Verification items for the finished model (mm, model axes). A direction names the side the tool comes from. Give positions to 0.01 mm unless a question says otherwise; leave off trailing zeros. Loops run counter-clockwise (first coordinate to the right, second up) from the corner with the lowest first, then second, coordinate; pieces in that order, holes last. Notation, with made-up numbers: (68, -22.75) -> (106, -22.75) arc R19 ccw to (106, -14.75) -> close; hole circle Ø7 at (-17.5, 3.5). An arc over 180 degrees is marked (long way). Answer in a Markdown table with one row per item. Add a question column.
Q1. Gauge pin test, flat ends, axial feed: P1, Ø1.5, axis at x = -2.5, y = 0.5, coming from the -Z side; P2, Ø1, axis at x = -10.5, z = 3.5, coming from the -Y side; P3, Ø1.5, axis at x = -10, z = 2, coming from the +Y side; P4, Ø2, axis at x = -14, z = 1.5, coming from the -Y side. Record the tip position at first contact, or that the pin passes through.
Q2. Material ranges on probe 1 along Z at (x, y) = (-2.5, 2.15); probe 2 along X at (y, z) = (-1.7, 3.5); probe 3 along Y at (x, z) = (-16, 0.7), recorded low to high.
Q3. Section check D-D on z = 0.9. Enter the section's corners in (x, y), and give its area (3 significant figures).
Q4. Section check B-B on y = 0.9. Enter the section's corners in (x, z), and give its area (3 significant figures).
Q5. Section check C-C on z = 3.1. Enter the section's corners in (x, y), and give its area (3 significant figures).
Q6. Release check for a two-part mould opening along X. For faces 3 (the face through (-8.35, -2.08, 0.99)), 4 (the face through (-16.37, 0.37, 0.99)), 5 (the face through (0, -2, 2)), 6 (the face through (-9, 0, 2)) record: pulls with the +X half, pulls with the -X half, needs draft (parallel to the pull), parting line crosses it, or undercut.
Q7. Section check A-A on x = 0. Enter the section's corners in (y, z), and give its area (3 significant figures).
Q8. Set-up check for faces 1 (the face through (2.77, -1.15, 2.42)), 2 (the face through (-17.25, 0.06, 0.99)): record each of +Z, -Z, +X, -X, +Y, -Y from which the full face is reachable in a straight line by a thin tool's end or side.
```python
from build123d import *

# Parameters (mm, degrees)
SKETCH_1_R      = 3
SKETCH_1_R_2    = 2
EXTRUDE_1_DEPTH = 4
SKETCH_1_3_R    = 0.5
EXTRUDE_2_DEPTH = 2


with BuildPart() as part:
    # Sketch 1 → Extrude 1 (new body)
    with BuildSketch(Plane.XY):
        Circle(SKETCH_1_R)
        Circle(SKETCH_1_R_2, mode=Mode.SUBTRACT)
    extrude(amount=EXTRUDE_1_DEPTH)

    # Sketch 1_3 → Extrude 2 (add)
    with BuildSketch(Plane.XY):
        with BuildLine():
            ThreePointArc((-16.133954801, 1.278385172), (-17.249996909, 0.038363404), (-16.139481346, -1.206610152))
            Line((-16.139481346, -1.206610152), (-0.334755231, -2.981264654))
            ThreePointArc((-0.334755231, -2.981264654), (-2.999992581, 0.006671881), (-0.321491523, 2.982724124))
            Line((-0.321491523, 2.982724124), (-16.133954801, 1.278385172))
        make_face()
        with Locations((-16, 0.035583454)):
            Circle(SKETCH_1_3_R, mode=Mode.SUBTRACT)
    extrude(amount=EXTRUDE_2_DEPTH)


solid = part.part
```
Taken from the geometry:
| question | item | result |
|---|---|---|
| 1 | P1 | stops at z = 0 |
| 1 | P2 | passes through |
| 1 | P3 | stops at y = 2.02 |
| 1 | P4 | stops at y = -1.56 |
| 2 | probe 1 | z = 0 to 2 |
| 2 | probe 2 | x = -2.47 to -1.05, 1.05 to 2.47 |
| 2 | probe 3 | y = -1.22 to -0.46, 0.54 to 1.29 |
| 3 | outline | (-16.14, -1.21) -> (-0.33, -2.98) arc R3 ccw (long way) to (-0.32, 2.98) -> (-16.13, 1.28) arc R1.25 ccw to start; hole circle Ø1 at (-16, 0.04); hole circle Ø4 at (0, 0) |
| 3 | area | 71.6 mm² |
| 4 | outline | (-16.9, 0) -> (-1.79, 0) -> (-1.79, 4) -> (-2.86, 4) -> (-2.86, 2) -> (-16.9, 2) -> close; (1.79, 0) -> (2.86, 0) -> (2.86, 4) -> (1.79, 4) -> close |
| 4 | area | 36.7 mm² |
| 5 | outline | circle Ø6 at (0, 0); hole circle Ø4 at (0, 0) |
| 5 | area | 15.7 mm² |
| 6 | face 3 | pulls with the -X half |
| 6 | face 4 | undercut |
| 6 | face 5 | undercut |
| 6 | face 6 | needs draft |
| 7 | outline | (-3, 0) -> (-2, 0) -> (-2, 4) -> (-3, 4) -> close; (2, 0) -> (3, 0) -> (3, 4) -> (2, 4) -> close |
| 7 | area | 8.00 mm² |
| 8 | face 1 | +Z |
| 8 | face 2 | +Z, -Z, -X |
